For this review, take the finished solid that the model builds, in its own axes (mm). A direction names the side the tool comes from. Coordinates: 2 decimals unless noted, no trailing zeros. Loops run counter-clockwise (first coordinate to the right, second up) from the corner with the lowest first, then second, coordinate; pieces in that order, holes last.
1. Take a section at C-C, the plane x = 5. Count the separate pieces of the cut face and the enclosed holes in it, then the cut area to 3 significant figures.
2. Clearance check with flat-ended pins moving along their axes: P1, Ø16, axis at y = 49, z = 16, coming from the -X side; P2, Ø23, axis at y = 83, z = 16, coming from the +X side; P3, Ø25, axis at x = 47.5, y = 41, coming from the -Z side; P4, Ø15.5, axis at x = 44.5, z = 50.5, coming from the +Y side. State where each tip first meets the part, or that it passes through.
3. Take a section at D-D, the plane x = 40.5. State the section outline as (y, z) points, then the cut area to 3 significant figures.
4. Machinability: for faces 1 (the face through (56.3, 57, 43)), 2 (the face through (40, 31.433, 50)), 3 (the face through (40, 49, 67.31)), 4 (the face through (40, 66.8, 50)), which of the approach directions +Z, -Z, +X, -X, +Y, -Y give a long, thin tool a straight path to every point of the face, cutting with its end or side? Answer none if there is none.
5. Take a section at B-B, the plane z = 51. State the section outline as (x, y) points.
6. Take a section at A-A, the plane y = 49. State the section outline as (x, z) points.
7. To check wall thickness, follow probe 1 along Z at (x, y) = (9, 16); probe 2 along X at (y, z) = (42.5, 28); probe 3 along Z at (x, y) = (31.5, 49). State the ranges of each line that lie inside material, in increasing order.
8. Mouldability with a two-part tool opening along Y and no side actions: class faces 5 (the face through (27.76, 46.83, 41.24)), 6 (the face through (40, 49, 33.437)), 7 (the face through (12, 100, 49)) as pulls with the +Y half, pulls with the -Y half, needs draft (parallel to the pull), parting line crosses it, or undercut.
```python
from build123d import *

# Parameters (mm, degrees)
F0_W     = 33
F0_H     = 34
F0_R     = 10
F0_H_2   = 33
F0_W_2   = 34
F1_DEPTH = 25
F2_W     = 35.366706574
F2_H     = 33.8733626366
F2_W_2   = 35.166706574
F2_H_2   = 33.6733626366
F2_R     = 10
F3_DEPTH = 56.3


# Not quite as in the source:
# - a feature names something its author has since deleted; it is built from what else it names


with BuildPart() as f1:
    # F0 (on Right) → F1 (new body)
    with BuildSketch(Plane.YZ):
        with Locations((16.5, 50)):
            Rectangle(F0_W, F0_H)
        with Locations((16, 51)):
            Circle(F0_R, mode=Mode.SUBTRACT)
        with Locations((16.5, 83.5)):
            Rectangle(F0_W, F0_H_2)
        with Locations((16, 84)):
            Circle(F0_R, mode=Mode.SUBTRACT)
        with Locations((50, 83.5)):
            Rectangle(F0_W_2, F0_H_2)
        with Locations((49, 84)):
            Circle(F0_R, mode=Mode.SUBTRACT)
        with Locations((16.5, 16.5)):
            Rectangle(F0_W, F0_H_2)
        with Locations((16, 16)):
            Circle(F0_R, mode=Mode.SUBTRACT)
        with Locations((50, 50)):
            Rectangle(F0_W_2, F0_H)
        with Locations((49, 51)):
            Circle(F0_R, mode=Mode.SUBTRACT)
        with Locations((50, 16.5)):
            Rectangle(F0_W_2, F0_H_2)
        with Locations((49, 16)):
            Circle(F0_R, mode=Mode.SUBTRACT)
        with Locations((83.5, 16.5)):
            Rectangle(F0_W, F0_H_2)
        with Locations((83, 16)):
            Circle(F0_R, mode=Mode.SUBTRACT)
        with Locations((83.5, 50)):
            Rectangle(F0_W, F0_H)
        with Locations((83, 51)):
            Circle(F0_R, mode=Mode.SUBTRACT)
        with Locations((83.5, 83.5)):
            Rectangle(F0_W, F0_H_2)
        with Locations((83, 84)):
            Circle(F0_R, mode=Mode.SUBTRACT)
    extrude(amount=F1_DEPTH)

    # F2 (on Right) → F3 (join)
    with BuildSketch(Plane.YZ):
        with Locations((49.116646713, 50.3734805703)):
            Rectangle(F2_W, F2_H)
        with Locations((49.116646713, 50.3734805703)):
            Rectangle(F2_W_2, F2_H_2, mode=Mode.SUBTRACT)
        with Locations((49.116646713, 50.3734805703)):
            Rectangle(F2_W_2, F2_H_2)
        with Locations((49, 51)):
            Circle(F2_R, mode=Mode.SUBTRACT)
    extrude(amount=F3_DEPTH)


solid = f1.part
```
Results list:
1. separate pieces: 1
1. enclosed holes: 9
1. area: 7,170 mm2
2. P1: passes through
2. P2: stops at x = 25
2. P3: stops at z = 33.44
2. P4: stops at y = 66.8
3. outline: (31.43, 33.44) - (66.8, 33.44) - (66.8, 67.31) - (31.43, 67.31) - close; hole circle Ø20 at (49, 51)
3. area: 884 mm2
4. face 1: +Z, -Z, +X, +Y, -Y
4. face 2: +Z, -Z, +X, -Y
4. face 3: +Z, +X, +Y, -Y
4. face 4: +Z, -Z, +X, +Y
5. outline: (0, 0) - (25, 0) - (25, 6) - (0, 6) - close; (0, 26) - (25, 26) - (25, 31.43) - (56.3, 31.43) - (56.3, 39) - (0, 39) - close; (0, 59) - (56.3, 59) - (56.3, 66.8) - (25, 66.8) - (25, 73) - (0, 73) - close; (0, 93) - (25, 93) - (25, 100) - (0, 100) - close
6. outline: (0, 0) - (25, 0) - (25, 6) - (0, 6) - close; (0, 26) - (25, 26) - (25, 33.44) - (56.3, 33.44) - (56.3, 41) - (0, 41) - close; (0, 61) - (56.3, 61) - (56.3, 67.31) - (25, 67.31) - (25, 74) - (0, 74) - close; (0, 94) - (25, 94) - (25, 100) - (0, 100) - close
7. probe 1: z = 0 to 6, 26 to 41, 61 to 74, 94 to 100
7. probe 2: x = 0 to 25
7. probe 3: z = 33.44 to 41, 61 to 67.31
8. face 5: undercut
8. face 6: needs draft
8. face 7: pulls with the +Y half
